Build history of the part. All positions in model axes, mm. Face numbers are marked on the shaded views. A direction names the side the tool comes from. Round coordinates to 2 decimals unless told otherwise and drop trailing zeros. Write each loop counter-clockwise with the first axis right and the second up, starting at its lowest first coordinate (ties: lowest second). Pieces come first, ordered by that corner, then holes.
Item 1: Mould opens along Y. For the marked faces 4, 5 and 6 say: +Y half, -Y half, draft (parallel to the pull), parting line (faces both ways), or undercut.
Item 2: Band-saw the part on A-A, the plane z = -7.25. Write the cut outline in (x, y).
Item 3: Drop flat-ended pins along their axis: pin 1 Ø3 at (x, z) = (6.5, -4.5) entering from -Y; pin 2 Ø3 at (x, z) = (6, -1.5) entering from +Y; pin 3 Ø1 at (y, z) = (-6.5, -1.5) entering from +X. Give the stop position or say it passes through.
Item 4: Wall check: probe 1 along X at (y, z) = (-2.75, -6); probe 2 along Y at (x, z) = (2.5, -3.75); probe 3 along X at (y, z) = (-1.5, -5.5). Give the ranges that are in metal, low to high.
Item 5: 3-axis set-ups, long thin cutter, end or side, ignore diameter. For the marked faces 1, 2 and 3: which of +Z, -Z, +X, -X, +Y, -Y reach the whole face in a straight line?
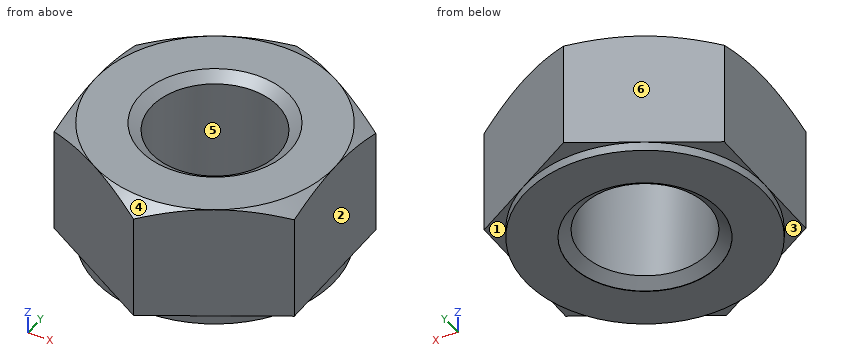
```python
from build123d import *

# Parameters (mm, degrees)
BASENUT_START = -8.4
BASENUTSKE_R  = 4.25
BASENUT_DEPTH = 8.4
SKETCH4_W     = 0.6
SKETCH4_H     = 11.237604307


# Read off the part's stored shape, not the designer's step: ThreadSchematic
with BuildPart() as part:
    # BaseNutSke → BaseNut (new body)
    with BuildSketch(Plane.XY.offset(BASENUT_START)):
        Polygon((8, 4.618802154), (8, -4.618802154), (0, -9.237604307), (-8, -4.618802154), (-8, 4.618802154), (0, 9.237604307), align=None)
        Circle(BASENUTSKE_R, mode=Mode.SUBTRACT)
    extrude(amount=BASENUT_DEPTH)

    # Sketch5 (on Front Plane) → EndChamfer (revolve, cut)
    with BuildSketch(Plane.XY):
        Polygon((8.3746, 5), (7.796928781, 4.175), (8.4254, 4.175), (8.4254, 5), align=None)
    revolve(axis=Axis((8.3746, 5, 0), (-0.5735764363510462, -0.8191520442889919, 0)), mode=Mode.SUBTRACT)

    # Sketch4 → Bearing-Face (revolve, cut)
    with BuildSketch(Plane(origin=(0, 0, 0), x_dir=(0, 0, -1), z_dir=(1, 0, 0)), mode=Mode.PRIVATE) as bearing_face_sk:
        with Locations((8.1, 13.618802154)):
            Rectangle(SKETCH4_W, SKETCH4_H)
        Polygon((0, 8), (-10, 8), (-10, 19.237604307), (0.71453118, 19.237604307), (0.71453118, 9.237604307), align=None)
    revolve(bearing_face_sk.sketch.rotate(Axis((0, 0, 0), (0, 0, -1)), 270), axis=Axis((0, 0, 0), (0, 0, -1)), mode=Mode.SUBTRACT)

    # ThreadSchematic outline → ThreadSchematic (revolve, cut)
    with BuildSketch(Plane.XZ):
        Polygon((4.25, 0), (4.25, -0.525155654), (5, 0), align=None)
        Polygon((5, -8.3746), (4.25, -7.849444346), (4.25, -8.4), (5, -8.4), align=None)
    revolve(axis=Axis((0, 0, 0), (0, 0, 1)), mode=Mode.SUBTRACT)


solid = part.part
```
Results:
1. face 4: -Y half
1. face 5: undercut
1. face 6: +Y half
2. outline: (-8, -4.62) - (0, -9.24) - (8, -4.62) - (8, 4.62) - (0, 9.24) - (-8, 4.62) - close; hole circle Ø8.5 at (0, 0)
3. pin 1: stops at y = -6.35
3. pin 2: stops at y = 6.64
3. pin 3: stops at x = 5.61
4. probe 1: x = -8 to -3.24, 3.24 to 8
4. probe 2: y = -7.79 to -3.44, 3.44 to 7.79
4. probe 3: x = -8 to -3.98, 3.98 to 8
5. face 1: -Z, +X, +Y
5. face 2: +Z, -Z, +X, +Y, -Y
5. face 3: -Z, -X, -Y
